from build123d import *

# Parameters (mm, degrees)
SKETCH_1_W          = 130
SKETCH_1_H          = 10
EXTRUDE_1_DEPTH     = 7
SKETCH_2_W          = 150
SKETCH_2_H          = 10
EXTRUDE_2_DEPTH     = 5
SKETCH_5_W          = 130
SKETCH_5_H          = 10
EXTRUDE_4_DEPTH     = 18
SKETCH_3_W          = 30
SKETCH_3_H          = 18
CUT_EXTRUDE_1_DEPTH = 4
SKETCH_6_W          = 5
SKETCH_6_H          = 10
EXTRUDE_5_DEPTH     = 10


with BuildPart() as part:
    # 스케치1 → 보스-돌출1 (new body)
    with BuildSketch(Plane.XY):
        Rectangle(SKETCH_1_W, SKETCH_1_H)
    extrude(amount=EXTRUDE_1_DEPTH)

    # 스케치2 → 보스-돌출2 (add)
    with BuildSketch(Plane(origin=(0, 0, 0), x_dir=(-1, 0, 0), z_dir=(0, 0, -1))):
        Rectangle(SKETCH_2_W, SKETCH_2_H)
    extrude(amount=EXTRUDE_2_DEPTH)

    # 스케치5 → 보스-돌출4 (add)
    with BuildSketch(Plane.XY.offset(7)):
        Rectangle(SKETCH_5_W, SKETCH_5_H)
    extrude(amount=EXTRUDE_4_DEPTH)

    # 스케치3 → 컷-돌출1 (cut)
    with BuildSketch(Plane(origin=(0, -5, 0), x_dir=(1, 0, 0), z_dir=(0, 1, 0))):
        with Locations((-44, -13)):
            Rectangle(SKETCH_3_W, SKETCH_3_H)
        with Locations((44, -13)):
            Rectangle(SKETCH_3_W, SKETCH_3_H)
    extrude(amount=CUT_EXTRUDE_1_DEPTH, mode=Mode.SUBTRACT)

    # 스케치6 → 보스-돌출5 (add)
    with BuildSketch(Plane.ZY.offset(65)):
        with Locations((9.5, 0)):
            Rectangle(SKETCH_6_W, SKETCH_6_H)
    extrude_5 = extrude(amount=EXTRUDE_5_DEPTH)

    # 대칭 복사1: 보스-돌출5 across plane
    add(extrude_5.mirror(Plane.ZY))


solid = part.part
The listing builds one solid part. Answer for the finished solid, in the listing's coordinates (mm). A direction names the side the tool comes from. Give positions to 0.01 mm unless a question says otherwise; leave off trailing zeros. Write each loop counter-clockwise with the first axis right and the second up, starting at its lowest first coordinate (ties: lowest second). Pieces come first, ordered by that corner, then holes.
1) Section C-C (z = 16) is taken. Write down the section's boundary in (x, y), and give its area (3 significant figures).
2) Find the intervals of material crossed by L1, parallel to Z at x = -67.5, y = -4; L2, parallel to Z at x = 36.5, y = -1.5; L3, parallel to Y at x = -48.5, z = 6.75, in increasing order.
3) Section B-B (z = 9.5) is taken. Write down the section's boundary in (x, y), and give its area (3 significant figures).
4) Section D-D (z = 1.5) is taken. Write down the section's boundary in (x, y).
5) Given P1, Ø1.5, axis at x = 42, z = 20, coming from the -Y side; P2, Ø3.5, axis at y = -2, z = 2.5, coming from the -X side; P3, Ø4.5, axis at y = -3.5, z = 16.5, coming from the +X side, each flat-ended and moving along its own axis, determine where each tip first touches the part or whether it passes through.
6) For a pull along Y with two mould halves and no side action, classify faces 5 (the face through (-1, 5, 10)), 6 (the face through (44, -1, 13)), 7 (the face through (-75, 0, 9)) as pulls with the +Y half, pulls with the -Y half, needs draft (parallel to the pull), parting line crosses it, or undercut.
7) Section A-A (y = -2.5) is taken. Write down the section's boundary in (x, z), and give its area (3 significant figures).
8) A tool of negligible diameter and unlimited length cuts with its end or side. For faces 1 (the face through (-44, -3, 22)), 2 (the face through (70, 0, 12)), 3 (the face through (-65, 0, 3)), 4 (the face through (70, 0, 7)), from which of +Z, -Z, +X, -X, +Y, -Y can it reach the whole face along a straight path? Write none if from no direction.
Response:
1. outline: (-65, -5) - (-59, -5) - (-59, -1) - (-29, -1) - (-29, -5) - (29, -5) - (29, -1) - (59, -1) - (59, -5) - (65, -5) - (65, 5) - (-65, 5) - close
1. area: 1,060 mm2
2. L1: z = -5 to 0, 7 to 12
2. L2: z = -5 to 4, 22 to 25
2. L3: y = -1 to 5
3. outline: (-75, -5) - (-59, -5) - (-59, -1) - (-29, -1) - (-29, -5) - (29, -5) - (29, -1) - (59, -1) - (59, -5) - (75, -5) - (75, 5) - (-75, 5) - close
3. area: 1,260 mm2
4. outline: (-65, -5) - (65, -5) - (65, 5) - (-65, 5) - close
5. P1: stops at y = -1
5. P2: stops at x = -65
5. P3: stops at x = 65
6. face 5: pulls with the +Y half
6. face 6: pulls with the -Y half
6. face 7: needs draft
7. outline: (-75, -5) - (75, -5) - (75, 0) - (65, 0) - (65, 7) - (75, 7) - (75, 12) - (65, 12) - (65, 25) - (-65, 25) - (-65, 12) - (-75, 12) - (-75, 7) - (-65, 7) - (-65, 0) - (-75, 0) - close; hole (-59, 4) - (-29, 4) - (-29, 22) - (-59, 22) - close; hole (29, 4) - (59, 4) - (59, 22) - (29, 22) - close
7. area: 3,020 mm2
8. face 1: -Y
8. face 2: +Z, +X, +Y, -Y
8. face 3: -X, +Y, -Y
8. face 4: +X, +Y, -Y
